from build123d import *

# Parameters (mm, degrees)
SALIENTE_EXTRUIR1_DEPTH                              = 20
TALADRO_DE_MARGEN_PARA_M31_D                         = 3
CHAFL_N2_SIZE                                        = 1
CROQUIS4_W                                           = 3
CROQUIS4_H                                           = 40
SALIENTE_EXTRUIR2_DEPTH                              = 6
AVELLANADO_PARA_TORNILLO_CON_CABEZA_OVAL_D           = 2.9
AVELLANADO_PARA_TORNILLO_CON_CABEZA_OVAL_CSINK_D     = 5.5
AVELLANADO_PARA_TORNILLO_CON_CABEZA_OVAL_CSINK_ANGLE = 90


with BuildPart() as part:
    # Croquis1 → Saliente-Extruir1 (new, symmetric)
    with BuildSketch(Plane(origin=(0, 0, 0), x_dir=(0, 1, 0), z_dir=(0, 0, 1))):
        Polygon((-6, 0), (6, 0), (6, 3), (4.5, 4.5), (4.5, 11.5), (2.5, 11.5), (2.5, 4.5), (-2.5, 4.5), (-2.5, 11.5), (-4.5, 11.5), (-4.5, 4.5), (-6, 3), align=None)
    extrude(amount=SALIENTE_EXTRUIR1_DEPTH, both=True)

    # Taladro de margen para M31 (through all)
    with Locations(Plane(origin=(0, 4.5, 0), x_dir=(-1, 0, 0), z_dir=(0, 1, 0))):
        with Locations((8, -10), (8, 10)):
            Hole(TALADRO_DE_MARGEN_PARA_M31_D / 2)

    # Chaflán2
    chafl_n2_edges = [part.edges().sort_by_distance(p)[0] for p in [
        (-11.5, -3.5, -20),
        (-11.5, 3.5, -20),
        (-11.5, 3.5, 20),
        (-11.5, -3.5, 20),
    ]]
    chamfer(chafl_n2_edges, length=CHAFL_N2_SIZE)

    # Croquis4 → Saliente-Extruir2 (add)
    with BuildSketch(Plane.XZ.offset(6)):
        with Locations((-1.5, 0)):
            Rectangle(CROQUIS4_W, CROQUIS4_H)
    extrude(amount=SALIENTE_EXTRUIR2_DEPTH)

    # Avellanado para tornillo con cabeza ovalada de M2.51 (through all)
    with Locations(Plane(origin=(-3, 0, 0), x_dir=(0, -1, 0), z_dir=(-1, 0, 0))):
        with Locations((9, 0)):
            CounterSinkHole(AVELLANADO_PARA_TORNILLO_CON_CABEZA_OVAL_D / 2, AVELLANADO_PARA_TORNILLO_CON_CABEZA_OVAL_CSINK_D / 2, counter_sink_angle=AVELLANADO_PARA_TORNILLO_CON_CABEZA_OVAL_CSINK_ANGLE)


solid = part.part
Model file for the job. Use its own axes, mm. A direction names the side the tool comes from. Give positions to 0.01 mm unless a question says otherwise; leave off trailing zeros. Loops run counter-clockwise (first coordinate to the right, second up) from the corner with the lowest first, then second, coordinate; pieces in that order, holes last.
1) Flat gauge pins, fed straight in: pin 1 Ø5 at (x, z) = (-8, -10) entering from -Y; pin 2 Ø5.5 at (x, z) = (-8.5, 1.5) entering from +Y; pin 3 Ø6 at (x, y) = (-9, -9) entering from +Z; pin 4 Ø5 at (y, z) = (-10, 5.5) entering from -X. Where does each tip first touch, or does it go through?
2) Saw through at A-A (z = 10). Write the cut outline in (x, y), plus the area to 4 significant figures.
3) Saw through at B-B (x = -2.5). Write the cut outline in (y, z).
4) Saw through at C-C (z = 0). Write the cut outline in (x, y), plus the area to 3 significant figures.
5) Saw through at D-D (x = -7). Write the cut outline in (y, z), plus the area to 3 significant figures.
6) Pull direction Z, two halves, no side cores. Call faces 4 (the cylindrical face through (-9.2, -3.5, 9.1)), 5 (the flat face through (-11.5, -3, 0)), 6 (the flat face through (-3, -1, 20)), 7 (the cylindrical face through (-0.84, -10.45, 0.06)): +Z half, -Z half, draft (parallel to the pull), parting line (faces both ways), or undercut.
7) Tool access for faces 1 (the flat face through (-8, -2.5, 0)), 2 (the flat face through (-8, 4.5, 0)), 3 (the flat face through (-3, -9, -5)): list every direction of +Z, -Z, +X, -X, +Y, -Y with a clear straight run to the whole face (end or side of a thin tool).
8) Wall check: line 1 (Z direction, x = -8, y = -4); line 2 (Y direction, x = -5, z = 6); line 3 (Z direction, x = -1.3, y = -9). Give the ranges that are in metal, low to high.
Answer block:
1. pin 1: stops at y = -4.5
1. pin 2: stops at y = 4.5
1. pin 3: passes through
1. pin 4: stops at x = -3
2. outline: (-11.5, -4.5) - (-9.5, -4.5) - (-9.5, -2.5) - (-11.5, -2.5) - close; (-11.5, 2.5) - (-9.5, 2.5) - (-9.5, 4.5) - (-11.5, 4.5) - close; (-6.5, -4.5) - (-4.5, -4.5) - (-3, -6) - (-3, -12) - (0, -12) - (0, 6) - (-3, 6) - (-4.5, 4.5) - (-6.5, 4.5) - (-6.5, 2.5) - (-4.5, 2.5) - (-4.5, -2.5) - (-6.5, -2.5) - close
2. area: 85.75 mm2
3. outline: (-12, -20) - (6, -20) - (6, 20) - (-12, 20) - close; hole circle Ø4.5 at (-9, 0)
4. outline: (-11.5, -4.5) - (-4.5, -4.5) - (-3, -6) - (-3, -6.25) - (-1.7, -7.55) - (0, -7.55) - (0, 6) - (-3, 6) - (-4.5, 4.5) - (-11.5, 4.5) - (-11.5, 2.5) - (-4.5, 2.5) - (-4.5, -2.5) - (-11.5, -2.5) - close; (-3, -12) - (0, -12) - (0, -10.45) - (-1.7, -10.45) - (-3, -11.75) - close
4. area: 87.4 mm2
5. outline: (-4.5, -20) - (-2.5, -20) - (-2.5, -11.12) - (-4.5, -11.12) - close; (-4.5, -8.88) - (-2.5, -8.88) - (-2.5, 8.88) - (-4.5, 8.88) - close; (-4.5, 11.12) - (-2.5, 11.12) - (-2.5, 20) - (-4.5, 20) - close; (2.5, -20) - (4.5, -20) - (4.5, -11.12) - (2.5, -11.12) - close; (2.5, -8.88) - (4.5, -8.88) - (4.5, 8.88) - (2.5, 8.88) - close; (2.5, 11.12) - (4.5, 11.12) - (4.5, 20) - (2.5, 20) - close
5. area: 142 mm2
6. face 4: undercut
6. face 5: draft
6. face 6: +Z half
6. face 7: undercut
7. face 1: +Z, -Z, -X
7. face 2: +Z, -Z, -X, +Y
7. face 3: +Z, -Z, -X, -Y
8. line 1: z = -20 to -11.5, -8.5 to 8.5, 11.5 to 20
8. line 2: y = -4.5 to -2.5, 2.5 to 4.5
8. line 3: z = -20 to -1.45, 1.45 to 20
